Study the drawing (mm; zero at the part's minimum x, y, z) and answer. A direction names the side the tool comes from. Give positions to 0.01 mm unless a question says otherwise; leave off trailing zeros. Write each loop counter-clockwise with the first axis right and the second up, starting at its lowest first coordinate (ties: lowest second). Pieces come first, ordered by that corner, then holes. Notation, with made-up numbers: (85.25, 21.25) - (98.25, 21.25) arc R26 cw to (98.25, 60.25) - close; hole circle Ø9 at (88, -9.75). An arc over 180 degrees is marked (long way). Return JSON: item names as keys, results as strings.
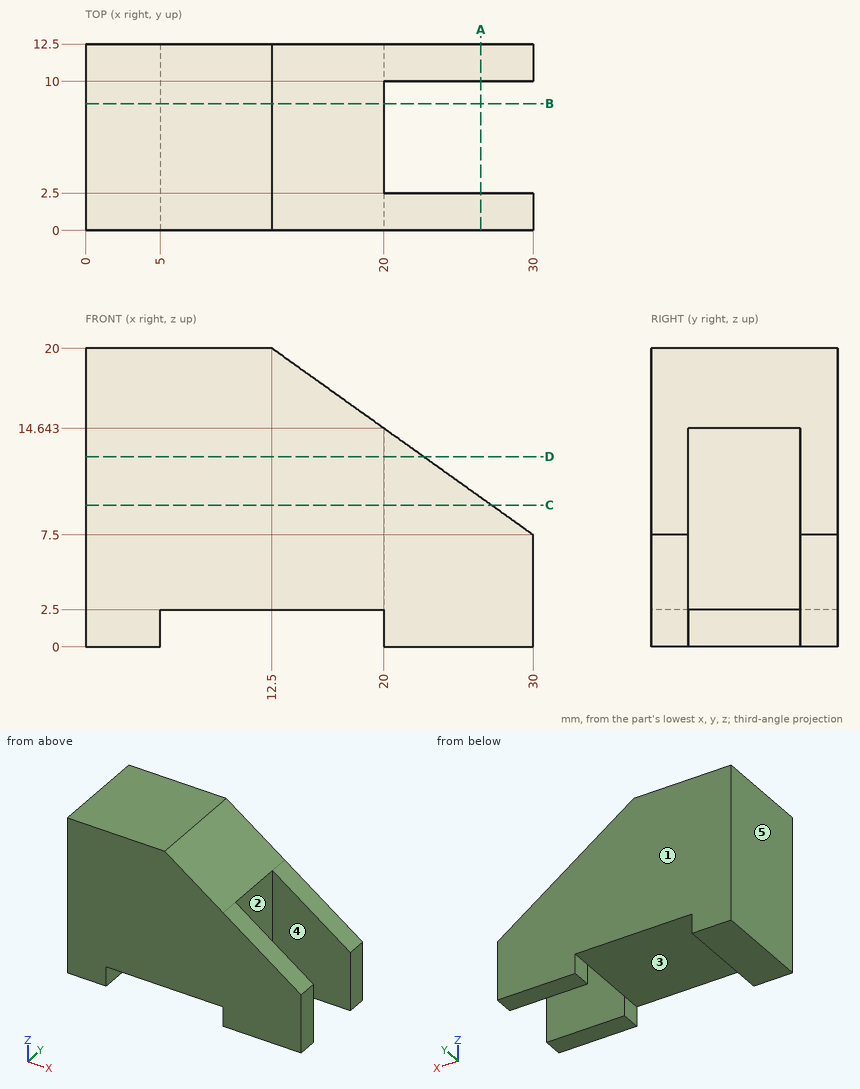
Item 1: Flat-ended cylindrical pins translate along their axes: P1, Ø3, axis at x = 27, z = 4, coming from the -Y side; P2, Ø4, axis at y = 7, z = 7, coming from the +X side; P3, Ø6, axis at x = 22.5, y = 10, coming from the +Z side. Find the tip coordinate at first contact, or state that the pin passes through.
Answer below:
{"P1": "stops at y = 0", "P2": "stops at x = 20", "P3": "stops at z = 15"}
Item 2: For the marked faces 4 and 5, determine the directions among +Z, -Z, +X, -X, +Y, -Y from which every point of the face is accessible in a straight line to the end or side of a thin tool.
Answer below:
{"face 4": "+Z, -Z, +X", "face 5": "+Z, -Z, -X, +Y, -Y"}
Item 3: Consider L1, parallel to X at y = 10.25, z = 1.25; L2, parallel to X at y = 6.5, z = 10.5; L3, parallel to X at y = 6, z = 2.25. Determine where each line is inside the solid, lowest interval first.
Answer below:
{"L1": "x = 0 to 5, 20 to 30", "L2": "x = 0 to 20", "L3": "x = 0 to 5"}
Item 4: The mould has two halves that part along X. Classify the marked faces 1, 2 and 3: +X half, -X half, draft (parallel to the pull), parting line (faces both ways), or undercut.
Answer below:
{"face 1": "draft", "face 2": "+X half", "face 3": "undercut"}
Item 5: A cutting plane is placed at D-D on z = 12.75. Determine the outline of the cut face in (x, y).
Answer below:
{"outline": "(0, 0) - (22.65, 0) - (22.65, 2.5) - (20, 2.5) - (20, 10) - (22.65, 10) - (22.65, 12.5) - (0, 12.5) - close"}
Item 6: A cutting plane is placed at C-C on z = 9.5. Determine the outline of the cut face in (x, y), then the cut area to 3 significant figures.
Answer below:
{"outline": "(0, 0) - (27.2, 0) - (27.2, 2.5) - (20, 2.5) - (20, 10) - (27.2, 10) - (27.2, 12.5) - (0, 12.5) - close", "area": "286 mm²"}
Item 7: A cutting plane is placed at A-A on x = 26.5. Determine the outline of the cut face in (y, z).
Answer below:
{"outline": "(0, 0) - (2.5, 0) - (2.5, 10) - (0, 10) - close; (10, 0) - (12.5, 0) - (12.5, 10) - (10, 10) - close"}
Item 8: A cutting plane is placed at B-B on y = 8.5. Determine the outline of the cut face in (x, z), then the cut area to 3 significant figures.
Answer below:
{"outline": "(0, 0) - (5, 0) - (5, 2.5) - (20, 2.5) - (20, 14.64) - (12.5, 20) - (0, 20) - close", "area": "342 mm²"}
